Design review of the part built by this model. Coordinates are the model's own, in mm. A direction names the side the tool comes from. Coordinates: 2 decimals unless noted, no trailing zeros. Write each loop counter-clockwise with the first axis right and the second up, starting at its lowest first coordinate (ties: lowest second). Pieces come first, ordered by that corner, then holes. Notation, with made-up numbers: M 49.5,23.5 L 106.5,23.5 A31 cw 106.5,47.5 Z; hole C 85,23.5 d2. An arc over 180 degrees is marked long. One line per question, with ' | ' between items.
from build123d import *

# Parameters (mm, degrees)
BOSS_EXTRUDE1_DEPTH = 2


with BuildPart() as part:
    # Sketch1 → Boss-Extrude1 (new, symmetric)
    with BuildSketch(Plane(origin=(0, 0, 0), x_dir=(1, 0, 0), z_dir=(0, 1, 0))):
        with BuildLine():
            Line((7.5, -30), (-7.5, -30))
            Line((-7.5, -30), (-7.5, -27.5))
            Line((-7.5, -27.5), (-5.75, -27.5))
            ThreePointArc((-5.75, -27.5), (-4.5, -26.25), (-5.75, -25))
            Line((-5.75, -25), (-34, -25))
            ThreePointArc((-34, -25), (-36.629076053, -25.606674578), (-38.726487571, -27.304013631))
            ThreePointArc((-38.726487571, -27.304013631), (-40.391401006, -28.070018299), (-41.981232738, -27.158352266))
            ThreePointArc((-41.981232738, -27.158352266), (0, 50), (41.981232738, -27.158352266))
            ThreePointArc((41.981232738, -27.158352266), (40.391401006, -28.070018299), (38.726487571, -27.304013631))
            ThreePointArc((38.726487571, -27.304013631), (36.629076053, -25.606674578), (34, -25))
            Line((34, -25), (5.75, -25))
            ThreePointArc((5.75, -25), (4.5, -26.25), (5.75, -27.5))
            Line((5.75, -27.5), (7.5, -27.5))
            Line((7.5, -27.5), (7.5, -30))
        make_face()
        with BuildLine():
            Line((21.071283391, 20.5), (-14.071283391, 20.5))
            ThreePointArc((-14.071283391, 20.5), (-16.073941577, 18.597333441), (-17.871710273, 16.5))
            Line((-17.871710273, 16.5), (-30, 16.5))
            Line((-30, 16.5), (-30, -7.5))
            Line((-30, -7.5), (-22.437424699, -7.5))
            ThreePointArc((-22.437424699, -7.5), (-19.204667359, -14.611573498), (-14.071283391, -20.5))
            Line((-14.071283391, -20.5), (21.071283391, -20.5))
            ThreePointArc((21.071283391, -20.5), (30.5, 0), (21.071283391, 20.5))
        make_face(mode=Mode.SUBTRACT)
    extrude(amount=BOSS_EXTRUDE1_DEPTH, both=True)


solid = part.part
1. Take a section at A-A (z = 0). Write out the cut boundary in (x, y).
Answer sheet:
outline: M -50,-2 L -30,-2 L -30,2 L -50,2 Z; M 30.5,-2 L 50,-2 L 50,2 L 30.5,2 Z
2. To check wall thickness, follow line 1 along X through (y, z) = (-0.2, 17.5); line 2 along X through (y, z) = (1.4, 9); line 3 along Z through (x, y) = (-16.5, -1.5). State the ranges of each line that lie inside material, in increasing order. Write a range as [from, to].
Answer sheet:
line 1: [-46.84, -17.06], [24.06, 46.84] | line 2: [-49.18, -21.96], [28.96, 49.18] | line 3: [-47.2, -18.14], [18.14, 25]
3. Draft analysis for pull direction Z (two halves, no side actions). For faces 1 (the face through (-4.5, 0, 26.3)), 2 (the face through (-7.5, 0, 29)), 3 (the face through (-1.501, 0.028, -49.977)), state which applies: pulls with the +Z half, pulls with the -Z half, needs draft (parallel to the pull), parting line crosses it, or undercut.
Answer sheet:
face 1: undercut | face 2: needs draft | face 3: parting line crosses it
4. Take a section at B-B (x = 0). Write out the cut boundary in (y, z).
Answer sheet:
outline: M -2,-50 L 2,-50 L 2,-20.5 L -2,-20.5 Z; M -2,20.5 L 2,20.5 L 2,30 L -2,30 Z
5. Tool access review of faces 4 (the face through (4.5, 0, 26.2)), 5 (the face through (36.66, 0.03, 25.62)), 6 (the face through (1, -2, -28)): name each direction out of +Z, -Z, +X, -X, +Y, -Y from which nothing blocks a thin tool from reaching the whole face with its end or side.
Answer sheet:
face 4: +Y, -Y | face 5: +Z, +Y, -Y | face 6: +Z, -Z, +X, -X, -Y
6. Take a section at D-D (z = -37). Write out the cut boundary in (x, y), then the cut area to 3 significant figures.
Answer sheet:
outline: M -33.63,-2 L 33.63,-2 L 33.63,2 L -33.63,2 Z | area: 269 mm^2
7. Take a section at C-C (y = -0.75). Write out the cut boundary in (x, z).
Answer sheet:
outline: M -41.98,27.16 A50 ccw long 41.98,27.16 A2 ccw 38.73,27.3 A6 cw 34,25 L 5.75,25 A1.25 cw 5.75,27.5 L 7.5,27.5 L 7.5,30 L -7.5,30 L -7.5,27.5 L -5.75,27.5 A1.25 cw -5.75,25 L -34,25 A6 cw -38.73,27.3 A2 ccw Z; hole M -30,-16.5 L -17.87,-16.5 A27 ccw -14.07,-20.5 L 21.07,-20.5 A27 ccw 21.07,20.5 L -14.07,20.5 A27 ccw -22.44,7.5 L -30,7.5 Z
8. Insertion check: pin 1 Ø12 at (x, z) = (-13, 4) entering from -Y; pin 2 Ø1.2 at (y, z) = (0, 29) entering from -X; pin 3 Ø1.2 at (x, y) = (6, 0.5) entering from -Z; pin 4 Ø1.2 at (x, y) = (-22, -1) entering from +Z. Each pin has a flat end and moves straight along its axis. Give the tip position at first contact, or say it passes through.
Answer sheet:
pin 1: through | pin 2: x = -7.5 | pin 3: z = -49.71 | pin 4: z = 25
